Build history of the part. All positions in model axes, mm. Face numbers are marked on the shaded views. Give positions to 0.01 mm unless a question says otherwise; leave off trailing zeros. Loops run counter-clockwise (first coordinate to the right, second up) from the corner with the lowest first, then second, coordinate; pieces in that order, holes last. Notation, with made-up numbers: M 2,-2 L 46,-2 A27 ccw 46,27 Z; hole C -3,23 d6. An arc over 180 degrees is marked long. Answer as a JSON object with one key per item and string values. Group by question number.
1. Drop flat-ended pins along their axis: pin 1 Ø2 at (y, z) = (-18, 33.5) entering from +X; pin 2 Ø1 at (y, z) = (-28, -36.5) entering from +X; pin 3 Ø5 at (y, z) = (-36.5, -33) entering from +X. Give the stop position or say it passes through.
2. Slice it at C-C (x = 30.5). List the corners of the cut face in (y, z), then the cut area to 4 significant figures.
3. Slice it at B-B (y = -32). List the corners of the cut face in (x, z), then the cut area to 3 significant figures.
4. Slice it at A-A (z = 42). List the corners of the cut face in (x, y).
5. Drill centre lines: line 1 along Z through (x, y) = (619, -5); line 2 along Y through (x, z) = (383.5, 0); line 3 along X through (y, z) = (-30, -15). Where is each one in solid material? Low to high. Write a range as [from, to].
6. Mould opens along Z. For the marked faces 1 and 2 say: released by +Z, released by -Z, zero draft, split by the parting line, or undercut.
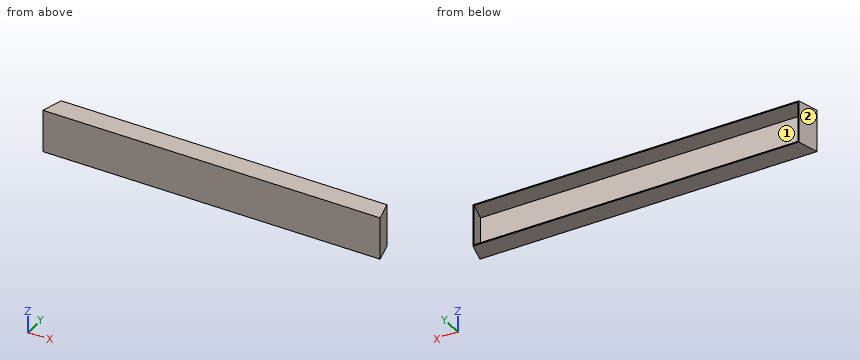
from build123d import *

# Parameters (mm, degrees)
F0_W     = 800
F0_H     = 100
F1_DEPTH = 50
F3_DEPTH = 100.001
F4_T     = -2.5


with BuildPart() as f1:
    # F0 (on Front) → F1 (new body)
    with BuildSketch(Plane.XZ):
        with Locations((337.88613, 1.85813)):
            Rectangle(F0_W, F0_H)
    extrude(amount=F1_DEPTH)

    # F2 (on face) → F3 (cut, through all)
    with BuildSketch(Plane.XY.offset(51.85813)):
        Polygon((-61.941713, -51.992044), (-62.11387, -50), (-36.069817, 47.197729), (-99.164672, 0), (-90.427369, -71.46059), align=None)
        Polygon((713.151226, 42.311921), (737.88613, -50), (805.342257, -50.860211), (814.011762, 33.620565), align=None)
    extrude(amount=-F3_DEPTH, mode=Mode.SUBTRACT)

    # F4
    f4_openings = [f1.faces().sort_by_distance(p)[0] for p in [
        (337.88613, 0, 1.85813),
    ]]
    offset(amount=F4_T, openings=f4_openings)


solid = f1.part
Established:
{
 "1": {"pin 1": "stops at x = 729.58", "pin 2": "stops at x = 732.13", "pin 3": "stops at x = 734.94"},
 "2": {"outline": "M -50,-48.14 L 0,-48.14 L 0,-45.64 L -47.5,-45.64 L -47.5,49.36 L 0,49.36 L 0,51.86 L -50,51.86 Z", "area": "487.5 mm^2"},
 "3": {"outline": "M -57.29,-48.14 L 733.06,-48.14 L 733.06,51.86 L -57.29,51.86 Z; hole M -54.7,-45.64 L 730.47,-45.64 L 730.47,49.36 L -54.7,49.36 Z", "area": "4,440 mm^2"},
 "4": {"outline": "M -62.11,-50 L 737.89,-50 L 724.49,0 L 721.9,0 L 734.63,-47.5 L -58.86,-47.5 L -46.13,0 L -48.72,0 Z"},
 "5": {"line 1": "z = [-48.14, -45.64], [49.36, 51.86]", "line 2": "y = [-50, -47.5]", "line 3": "x = [-56.75, -54.17], [729.94, 732.53]"},
 "6": {"face 1": "undercut", "face 2": "zero draft"}
}
